from build123d import *

# Parameters (mm, degrees)
BOSS_EXTRUDE1_DEPTH = 45
BOSS_EXTRUDE2_DEPTH = 35
SKETCH2_R           = 1.75
CUT_EXTRUDE1_DEPTH  = 4.55
CUT_EXTRUDE2_REACH  = 4
SKETCH3_R           = 1.75


with BuildPart() as part:
    # Sketch1 → Boss-Extrude1 (new body)
    with BuildSketch(Plane.XY):
        Polygon((0, 0), (0, 2), (10, 2), (10, 12), (11, 12), (11, 2), (12.55, 2), (12.55, 12), (13.55, 12), (13.55, 0), align=None)
    extrude(amount=BOSS_EXTRUDE1_DEPTH)

    # Sketch4 → Boss-Extrude2 (add)
    with BuildSketch(Plane.XY):
        Polygon((0, 2), (0, 0), (13.55, 0), (13.55, 3), (12.55, 3), (12.55, 2), (11, 2), (11, 3), (10, 3), (10, 2), align=None)
    extrude(amount=-BOSS_EXTRUDE2_DEPTH)

    # Sketch2 → Cut-Extrude1 (cut, through all)
    with BuildSketch(Plane.ZY.offset(-10)):
        with Locations((40, 7)):
            Circle(SKETCH2_R)
        with Locations((10, 7)):
            Circle(SKETCH2_R)
    extrude(amount=-CUT_EXTRUDE1_DEPTH, mode=Mode.SUBTRACT)

    # Sketch3 → Cut-Extrude2 (cut, up to next)
    with BuildSketch(Plane(origin=(0, 2, 0), x_dir=(1, 0, 0), z_dir=(0, 1, 0)), mode=Mode.PRIVATE) as cut_extrude2_sk1:
        with Locations((5, 25)):
            Circle(SKETCH3_R)
    cut_extrude2_tool1 = extrude(cut_extrude2_sk1.sketch, amount=-CUT_EXTRUDE2_REACH, mode=Mode.PRIVATE) & part.part
    add(cut_extrude2_tool1.solids().sort_by_distance((5, 2, -25))[0], mode=Mode.SUBTRACT)
    # Sketch3 → Cut-Extrude2 (cut, up to next)
    with BuildSketch(Plane(origin=(0, 2, 0), x_dir=(1, 0, 0), z_dir=(0, 1, 0)), mode=Mode.PRIVATE) as cut_extrude2_sk2:
        with Locations((5, -35)):
            Circle(SKETCH3_R)
    cut_extrude2_tool2 = extrude(cut_extrude2_sk2.sketch, amount=-CUT_EXTRUDE2_REACH, mode=Mode.PRIVATE) & part.part
    add(cut_extrude2_tool2.solids().sort_by_distance((5, 2, 35))[0], mode=Mode.SUBTRACT)


solid = part.part
Can you work these out from the model? Positions are in its coordinate system, mm. A direction names the side the tool comes from. Coordinates: 2 decimals unless noted, no trailing zeros. Loops run counter-clockwise (first coordinate to the right, second up) from the corner with the lowest first, then second, coordinate; pieces in that order, holes last. Notation, with made-up numbers: M 15.25,28.25 L 60.25,28.25 A30 cw 60.25,59.25 Z; hole C -19,60 d5. An arc over 180 degrees is marked long. Return JSON: item names as keys, results as strings. Group by question number.
Item 1: If I drill on L1, parallel to Z at x = 5, y = 0.9; L2, parallel to X at y = 9.25, z = 26; L3, parallel to X at y = 0.5, z = -25, over which ranges is the centre line in solid material (lowest first)? Write a range as from..to.
Item 2: Imagine slicing it at D-D (z = -13). Please give me the cut outline in (x, y).
Item 3: Imagine slicing it at C-C (x = 5). Please give me the cut outline in (y, z).
Item 4: Imagine slicing it at B-B (y = 7). Please give me the cut outline in (x, z), and give its area (3 significant figures).
Item 5: On a 3-axis mill with a long thin cutter (end or side, diameter ignored), from which of +Z, -Z, +X, -X, +Y, -Y can I reach the whole of each face in a straight line? I mean faces 5 (the flat face through (13.55, 5, 14)), 6 (the flat face through (12.55, 7, 14)), 7 (the flat face through (5, 2, 6)). Say none if no direction works.
Item 6: I'm going to push flat-ended pins straight in: pin 1 Ø8 at (x, z) = (6.5, 17.5) entering from +Y; pin 2 Ø4 at (y, z) = (7, 10) entering from -X; pin 3 Ø3 at (x, z) = (5, 35) entering from +Y; pin 4 Ø5.5 at (x, z) = (5, -25) entering from +Y. Where does each tip first touch, or does it pass through?
Item 7: Thinking about a two-plate mould opening in Y: for faces 1 (the cylindrical face through (3.25, 1.01, 34.92)), 2 (the cylindrical face through (10.49, 5.45, 10.81)), 3 (the flat face through (12, 2, 6)), 4 (the flat face through (7, 0, 6)), which applies, released by +Y, released by -Y, zero draft, split by the parting line, or undercut?
Item 8: Imagine slicing it at A-A (z = 40). Please give me the cut outline in (x, y).
Verdict:
{
 "1": {"L1": "z = -35..-26.75, -23.25..33.25, 36.75..45", "L2": "x = 10..11, 12.55..13.55", "L3": "x = 0..3.25, 6.75..13.55"},
 "2": {"outline": "M 0,0 L 13.55,0 L 13.55,3 L 12.55,3 L 12.55,2 L 11,2 L 11,3 L 10,3 L 10,2 L 0,2 Z"},
 "3": {"outline": "M 0,-35 L 2,-35 L 2,-26.75 L 0,-26.75 Z; M 0,-23.25 L 2,-23.25 L 2,33.25 L 0,33.25 Z; M 0,36.75 L 2,36.75 L 2,45 L 0,45 Z"},
 "4": {"outline": "M 10,0 L 11,0 L 11,8.25 L 10,8.25 Z; M 10,11.75 L 11,11.75 L 11,38.25 L 10,38.25 Z; M 10,41.75 L 11,41.75 L 11,45 L 10,45 Z; M 12.55,0 L 13.55,0 L 13.55,8.25 L 12.55,8.25 Z; M 12.55,11.75 L 13.55,11.75 L 13.55,38.25 L 12.55,38.25 Z; M 12.55,41.75 L 13.55,41.75 L 13.55,45 L 12.55,45 Z", "area": "76.0 mm^2"},
 "5": {"face 5": "+Z, -Z, +X, +Y, -Y", "face 6": "+Z, -Z, +Y", "face 7": "+Z, -Z, -X, +Y"},
 "6": {"pin 1": "stops at y = 12", "pin 2": "stops at x = 10", "pin 3": "passes through", "pin 4": "stops at y = 2"},
 "7": {"face 1": "zero draft", "face 2": "undercut", "face 3": "released by +Y", "face 4": "released by -Y"},
 "8": {"outline": "M 0,0 L 13.55,0 L 13.55,5.25 L 12.55,5.25 L 12.55,2 L 11,2 L 11,5.25 L 10,5.25 L 10,2 L 0,2 Z; M 10,8.75 L 11,8.75 L 11,12 L 10,12 Z; M 12.55,8.75 L 13.55,8.75 L 13.55,12 L 12.55,12 Z"}
}
